Input: part model. Units: mm. Frame: model coordinates. Give positions to 0.01 mm unless a question says otherwise; leave off trailing zeros. Loops run counter-clockwise (first coordinate to the right, second up) from the corner with the lowest first, then second, coordinate; pieces in that order, holes last. Notation, with made-up numbers: (-21, 35) -> (-1, 35) arc R11 ccw to (-1, 42) -> close; hole circle Ø7 at (61.5, 40.25). An arc over 180 degrees is marked (long way). Use CSV: the item, a comma, the result in double quotes.
```python
from build123d import *

# Parameters (mm, degrees)
RESSALTO_EXTRUS_O1_DEPTH = 12.26


with BuildPart() as part:
    # Esboço1 → Ressalto-extrusão1 (new body)
    with BuildSketch(Plane(origin=(0, 0, 0), x_dir=(1, 0, 0), z_dir=(0, 1, 0))):
        with BuildLine():
            Line((11.823645173, -27.571750304), (12.993920826, -30.334106573))
            Line((12.993920826, -30.334106573), (20.795690346, -48.749654144))
            ThreePointArc((20.795690346, -48.749654144), (24.072464244, -50.130779062), (25.453589161, -46.854005164))
            Line((25.453589161, -46.854005164), (25.198608413, -46.380200094))
            Line((25.198608413, -46.380200094), (15.823293166, -28.958995034))
            ThreePointArc((15.823293166, -28.958995034), (21.396881696, -25.123165678), (26.071005915, -20.231229586))
            ThreePointArc((26.071005915, -20.231229586), (26.997061933, -18.977846216), (27.862912529, -17.68214086))
            ThreePointArc((27.862912529, -17.68214086), (31.468158773, 9.937554199), (12.654282119, 30.477354611))
            ThreePointArc((12.654282119, 30.477354611), (3.9115652, 32.767356587), (-5.124534224, 32.599680198))
            Line((-5.124534224, 32.599680198), (-6.211556636, 39.514763876))
            ThreePointArc((-6.211556636, 39.514763876), (-21.202255924, 33.9184956), (-32.800073698, 22.894435249))
            Line((-32.800073698, 22.894435249), (-28.26846637, 17.015835516))
            Line((-28.26846637, 17.015835516), (-26.290601135, 14.450062005))
            ThreePointArc((-26.290601135, 14.450062005), (22.221192163, 20.154865886), (11.823645173, -27.571750304))
        make_face()
    extrude(amount=RESSALTO_EXTRUS_O1_DEPTH)


solid = part.part
```
1) Contact query for flat-ended pins moving along their axis: pin 1 (1.5 mm diameter, centred on y = 8.5, z = -7, fed in from -X); pin 2 (1.5 mm diameter, centred on y = 5, z = 29, fed in from -X); pin 3 (2 mm diameter, centred on x = -11.5, y = 7.5, fed in from -Z); pin 4 (5 mm diameter, centred on x = 26, z = 3, fed in from -Y). Output: stop coordinate, or through.
From the geometry:
pin 1,"stops at x = 28.98"
pin 2,"stops at x = 12.11"
pin 3,"stops at z = -38.6"
pin 4,"passes through"
2) Section query C-C (x = 0). Return loops of the section in (y, z), then the cut area to 3 significant figures.
From the geometry:
outline,"(0, -33) -> (12.26, -33) -> (12.26, -30) -> (0, -30) -> close"
area,"36.8 mm^2"
3) Section query B-B (z = -20). Return loops of the section in (x, y).
From the geometry:
outline,"(-30.57, 0) -> (-22.36, 0) -> (-22.36, 12.26) -> (-30.57, 12.26) -> close; (22.36, 0) -> (26.25, 0) -> (26.25, 12.26) -> (22.36, 12.26) -> close"
4) Section query A-A (y = 8.5). Return loops of the section in (x, z), then the cut area to 3 significant figures.
From the geometry:
outline,"(-32.8, -22.89) arc R40 ccw to (-6.21, -39.51) -> (-5.12, -32.6) arc R33 ccw to (15.82, 28.96) -> (25.45, 46.85) arc R2.51 ccw to (20.8, 48.75) -> (11.82, 27.57) arc R30 cw (long way) to (-26.29, -14.45) -> close"
area,"663 mm^2"
5) Mould query, pull axis Z, two halves, no side actions, for faces 1 (the flat face through (-5.66, 6.04, -36.01)), 2 (the cylindrical face through (21.677, 6.044, -20.739)), 3 (the flat face through (17, 12.26, -25)). Classes: pulls with the +Z half, pulls with the -Z half, needs draft (parallel to the pull), parting line crosses it, or undercut.
From the geometry:
face 1,"pulls with the -Z half"
face 2,"undercut"
face 3,"needs draft"
6) Section query D-D (z = 0). Return loops of the section in (x, y), then the cut area to 3 significant figures.
From the geometry:
outline,"(30, 0) -> (33, 0) -> (33, 12.26) -> (30, 12.26) -> close"
area,"36.8 mm^2"
7) Ray query, line 1 (Z direction, x = 23.5, y = 3.5); line 2 (X direction, y = 5, z = 0); line 3 (Z direction, x = 26, y = 5). Return the intervals inside material, ascending.
From the geometry:
line 1,"z = -23.17 to -18.65, 18.65 to 23.17, 43.22 to 50.29"
line 2,"x = 30 to 33"
line 3,"z = -20.32 to -14.97, 14.97 to 20.32"
